Source: three-view drawing plus pictorial views. Frame: mm from the lowest corner of the part. Give positions to 0.01 mm unless a question says otherwise; leave off trailing zeros. Write each loop counter-clockwise with the first axis right and the second up, starting at its lowest first coordinate (ties: lowest second). Pieces come first, ordered by that corner, then holes. Notation, with made-up numbers: (75.5, 17) -> (118.5, 17) arc R23 cw to (118.5, 35) -> close; hole circle Ø11 at (10.25, 17.25). An arc over 180 degrees is marked (long way). Answer in a Markdown table with one row per item. Add a question column.
Item 1: Section query B-B on y = 41. Output: boundary loops of the cut face in (x, z).
Item 2: First-contact query: P1, Ø1, axis at x = 227.5, z = 47.5, coming from the -Y side; P2, Ø8, axis at x = 202, z = 30.5, coming from the -Y side (1 decimal); P3, Ø10.5, axis at x = 139.5, y = 186, coming from the +Z side. Flat tips, straight axial feed; report the tip coordinate or a pass-through.
Item 3: Section query A-A on x = 134.5. Output: boundary loops of the cut face in (y, z) (1 decimal), plus the area to 3 significant figures.
Item 4: Section query C-C on z = 49. Output: boundary loops of the cut face in (x, y).
Item 5: Material intervals for probe 1 along Z at (x, y) = (192, 185); probe 2 along Z at (x, y) = (183, 162.5) (1 decimal); probe 3 along Z at (x, y) = (179, 161), sorted ascending. Write a range as from..to.
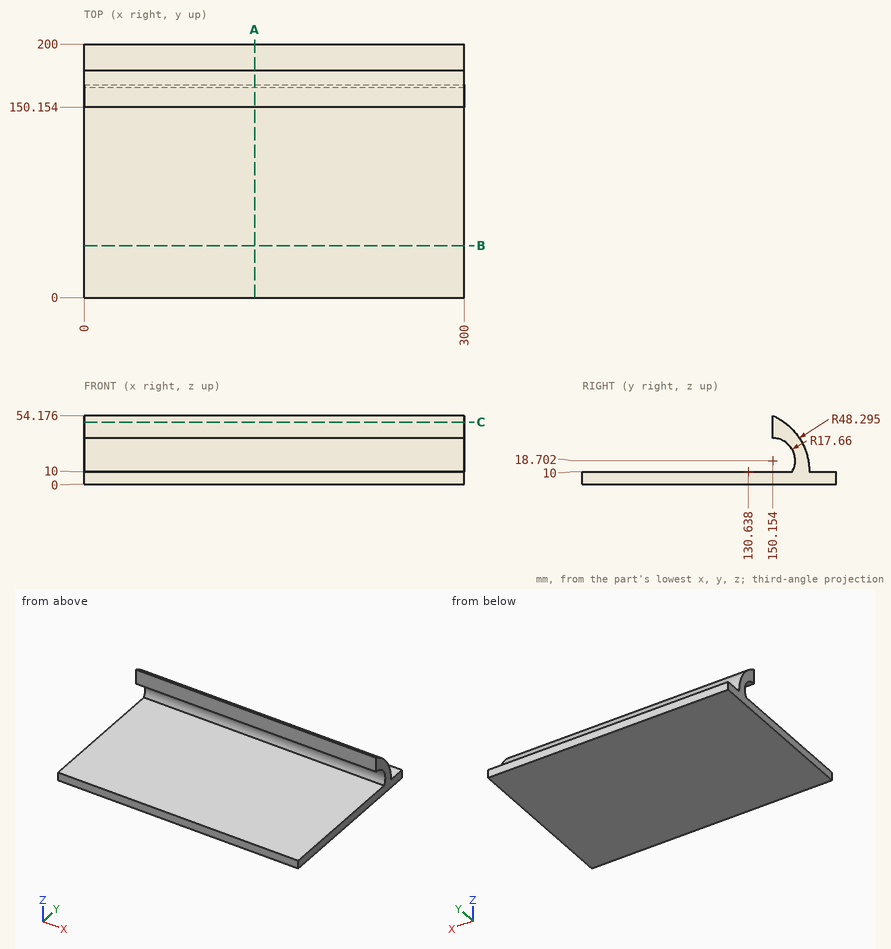
Findings below:
| question | item | result |
|---|---|---|
| 1 | outline | (0, 0) -> (300, 0) -> (300, 10) -> (0, 10) -> close |
| 2 | P1 | stops at y = 150.15 |
| 2 | P2 | stops at y = 158 |
| 2 | P3 | stops at z = 10 |
| 3 | outline | (0, 0) -> (200, 0) -> (200, 10) -> (178.9, 10) arc R48.3 ccw to (150.2, 54.2) -> (150.2, 36.4) arc R17.7 cw to (165.5, 10) -> (0, 10) -> close |
| 3 | area | 2,520 mm^2 |
| 4 | outline | (0, 150.15) -> (300, 150.15) -> (300, 159.12) -> (0, 159.12) -> close |
| 5 | probe 1 | z = 0..10 |
| 5 | probe 2 | z = 0..10, 31.3..46.3 |
| 5 | probe 3 | z = 0..10, 32.64..47.56 |
